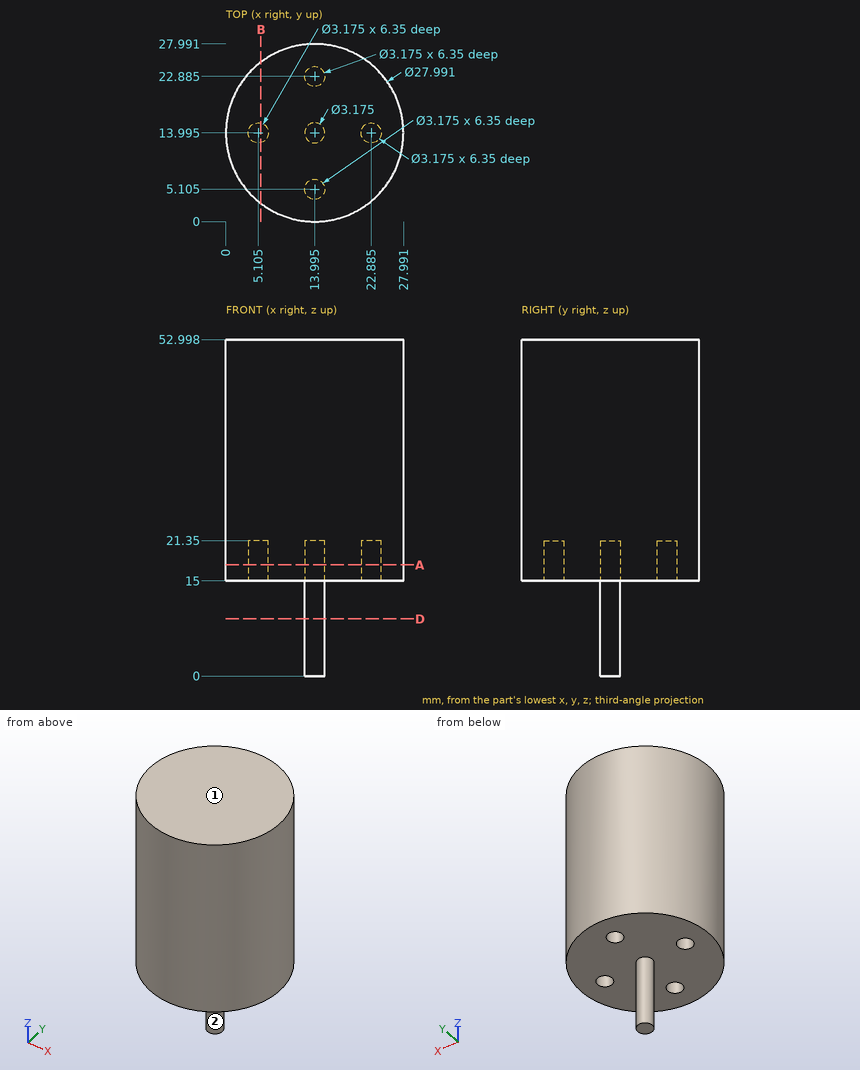
Geometry: see drawing. Coordinates: mm, zero at the bounding-box minimum. A direction names the side the tool comes from. Coordinates: 2 decimals unless noted, no trailing zeros. Loops run counter-clockwise (first coordinate to the right, second up) from the corner with the lowest first, then second, coordinate; pieces in that order, holes last.
Q1. Cut plane D-D (z = 9). Output: boundary loops of the cut face in (x, y) (1 decimal).
Q2. Set-up query: the marked faces 1 and 2. Return all of +Z, -Z, +X, -X, +Y, -Y with unobstructed straight access to the full face (end or side cutting, diameter ignored); none if empty.
Q3. Cut plane A-A (z = 17.5). Output: boundary loops of the cut face in (x, y) (1 decimal).
Q4. Material intervals for line 1 (Z direction, x = 10, y = 10.5); line 2 (X direction, y = 14.5, z = 33.5); line 3 (X direction, y = 25.75, z = 51), sorted ascending.
Q5. Cut plane B-B (x = 5.5). Output: boundary loops of the cut face in (y, z).
Q6. Contact query for flat-ended pins moving along their axis: pin 1 (10 mm diameter, centred on x = 3.5, z = 43.5, fed in from +Y); pin 2 (3.5 mm diameter, centred on x = 23, y = 14, fed in from -Z); pin 3 (1.6 mm diameter, centred on x = 14, y = 23.5, fed in from -Z). Output: stop coordinate, or through.
Working result:
1. outline: circle Ø3.2 at (14, 14)
2. face 1: +Z, +X, -X, +Y, -Y
2. face 2: -Z
3. outline: circle Ø28 at (14, 14); hole circle Ø3.2 at (5.1, 14); hole circle Ø3.2 at (14, 5.1); hole circle Ø3.2 at (14, 22.9); hole circle Ø3.2 at (22.9, 14)
4. line 1: z = 15 to 53
4. line 2: x = 0.01 to 27.98
4. line 3: x = 6.4 to 21.59
5. outline: (2.87, 15) - (12.46, 15) - (12.46, 21.35) - (15.53, 21.35) - (15.53, 15) - (25.12, 15) - (25.12, 53) - (2.87, 53) - close
6. pin 1: stops at y = 26.87
6. pin 2: stops at z = 15
6. pin 3: stops at z = 21.35
